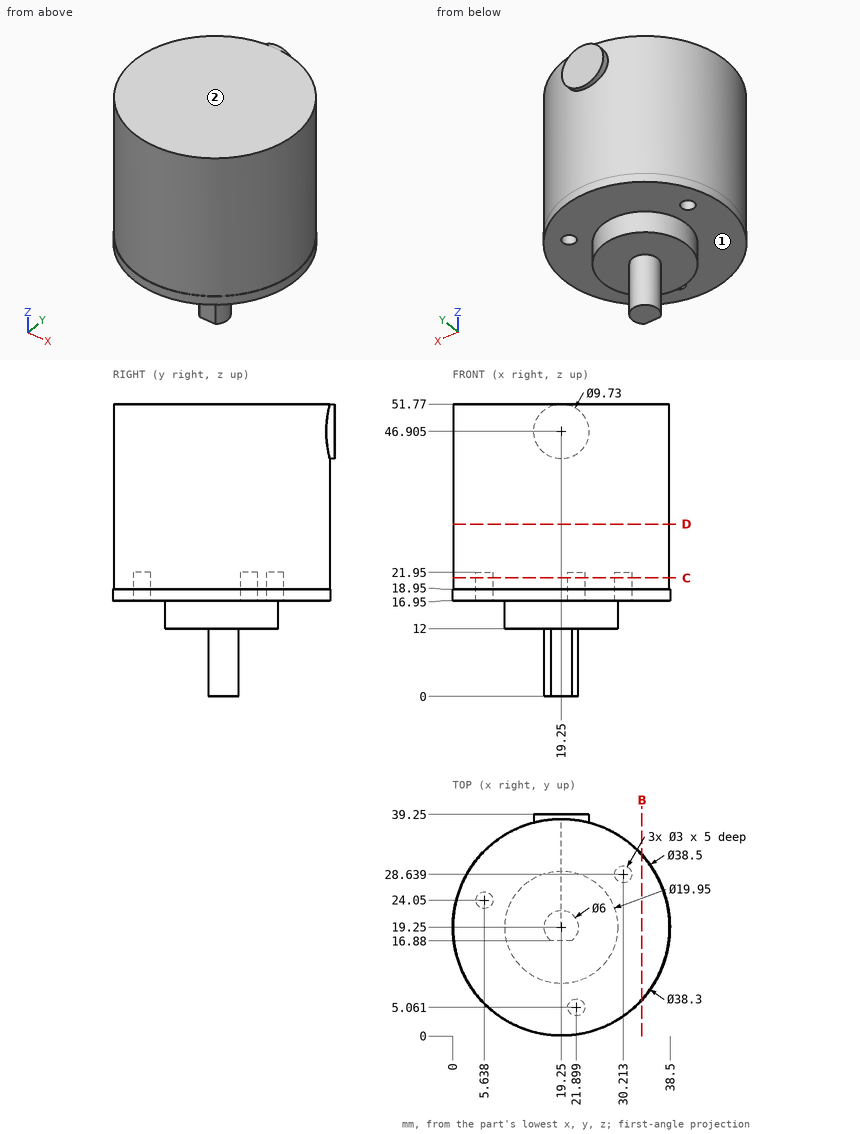
Part print with two shaded views. Sizes in mm from the minimum x, y, z corner. A direction names the side the tool comes from. Round coordinates to 2 decimals unless told otherwise and drop trailing zeros. Write each loop counter-clockwise with the first axis right and the second up, starting at its lowest first coordinate (ties: lowest second). Pieces come first, ordered by that corner, then holes. Notation, with made-up numbers: M -2,21 L 52,21 A17 cw 52,49 Z; hole C 2,29 d9. An arc over 180 degrees is marked long. Put each result on its own line as item: value. Start each with the question number.
1) Saw through at D-D, the plane z = 30.5. Write the cut outline in (x, y), and give its area (3 significant figures).
2) 3-axis set-ups, long thin cutter, end or side, ignore diameter. For the marked faces 1 and 2: which of +Z, -Z, +X, -X, +Y, -Y reach the whole face in a straight line?
3) Drill centre lines: probe 1 along Z at (x, y) = (30, 34); probe 2 along Z at (x, y) = (14, 13); probe 3 along Y at (x, z) = (6, 44) (1 decimal). Where is each one in solid material? Low to high. Write a range as [from, to].
4) Saw through at B-B, the plane x = 33.5. Write the cut outline in (y, z).
5) Saw through at C-C, the plane z = 21. Write the cut outline in (x, y).
6) Pin check, flat tips, straight feed: pin 1 Ø4 at (x, z) = (9.5, 23.5) entering from +Y; pin 2 Ø4 at (y, z) = (25, 46) entering from -X; pin 3 Ø2.5 at (x, y) = (30, 29.5) entering from -Z; pin 4 Ø2 at (y, z) = (7.5, 11.5) entering from +X. Stop position of each tip, or through.
Resolved:
1. outline: C 19.25,19.25 d38.3
1. area: 1,150 mm²
2. face 1: -Z
2. face 2: +Z, +X, -X, +Y, -Y
3. probe 1: [16.95, 51.77]
3. probe 2: [12, 51.77]
3. probe 3: [5.4, 33.1]
4. outline: M 6.31,16.95 L 32.19,16.95 L 32.19,18.95 L 32.04,18.95 L 32.04,51.77 L 6.46,51.77 L 6.46,18.95 L 6.31,18.95 Z
5. outline: C 19.25,19.25 d38.3; hole C 5.64,24.05 d3; hole C 21.9,5.06 d3; hole C 30.21,28.64 d3
6. pin 1: y = 36.76
6. pin 2: x = 0.47
6. pin 3: z = 16.95
6. pin 4: through
